from build123d import *

# Parameters (mm, degrees)
F0_W     = 7
F0_H     = 7
F0_W_2   = 4.5
F0_H_2   = 4.5
F1_DEPTH = 5
F2_W     = 7
F2_H     = 7
F3_DEPTH = 2
F4_W     = 1.960302
F4_H     = 7
F5_DEPTH = 15
F6_R     = 1.25
F7_DEPTH = 25


with BuildPart() as f1:
    # F0 (on Front) → F1 (new body)
    with BuildSketch(Plane.XZ):
        Rectangle(F0_W, F0_H)
        Rectangle(F0_W_2, F0_H_2, mode=Mode.SUBTRACT)
    extrude(amount=F1_DEPTH)

    # F2 (on face) → F3 (join)
    with BuildSketch(Plane.XZ.offset(5)):
        Rectangle(F2_W, F2_H)
    extrude(amount=F3_DEPTH)

    # F4 (on face) → F5 (join)
    with BuildSketch(Plane.XZ.offset(7)):
        Rectangle(F4_W, F4_H)
    extrude(amount=F5_DEPTH)

    # F6 (on face) → F7 (cut)
    with BuildSketch(Plane(origin=(-0.980151, 0, 0), x_dir=(0, -1, 0), z_dir=(-1, 0, 0))):
        with Locations((19, 0)):
            Circle(F6_R)
    extrude(amount=-F7_DEPTH, mode=Mode.SUBTRACT)


solid = f1.part
Work out the finished part from the listing and answer in its coordinate system (mm). A direction names the side the tool comes from. Give positions to 0.01 mm unless a question says otherwise; leave off trailing zeros. Write each loop counter-clockwise with the first axis right and the second up, starting at its lowest first coordinate (ties: lowest second). Pieces come first, ordered by that corner, then holes. Notation, with made-up numbers: (88, 46.25) - (147, 46.25) arc R28 ccw to (147, 64.25) - close; hole circle Ø9 at (34, -39.75). An arc over 180 degrees is marked (long way). One line per item, written item: value. Start each with the question number.
1. Find section C-C (x = 0.75). Write down the section's boundary in (y, z).
2. Find section D-D (z = 0). Write down the section's boundary in (x, y), then the cut area to 3 significant figures.
3. For a pull along X with two mould halves and no side action, classify faces 5 (the flat face through (0, -2, 2.25)), 6 (the cylindrical face through (-0.014, -20.155, -0.479)), 7 (the flat face through (3.5, -3, 0)) as +X half, -X half, draft (parallel to the pull), parting line (faces both ways), or undercut.
4. Find section B-B (y = -19). Write down the section's boundary in (x, z), then the cut area to 3 significant figures.
5. For faces 1 (the flat face through (0, -22, 0)), 2 (the flat face through (0.98, -14, 0)), 3 (the flat face through (0, -2, -2.25)), 4 (the flat face through (-2, -7, 0)), determine the directions among +Z, -Z, +X, -X, +Y, -Y from which every point of the face is accessible in a straight line to the end or side of a thin tool.
6. Given pin 1 (3 mm diameter, centred on x = 2, z = 0, fed in from -Y); pin 2 (1.5 mm diameter, centred on y = -13, z = 0, fed in from +X); pin 3 (2 mm diameter, centred on x = -2.5, z = 0, fed in from -Y), each flat-ended and moving along its own axis, determine where each tip first touches the part or whether it passes through.
7. Find section A-A (z = -1). Write down the section's boundary in (x, y), then the cut area to 3 significant figures.
8. Consider probe 1 along Z at (x, y) = (0.25, -19); probe 2 along Z at (x, y) = (1.75, -4.5); probe 3 along X at (y, z) = (-15.5, 2.5). Determine where each line is inside the solid, lowest interval first.
Geometry results:
1. outline: (-22, -3.5) - (0, -3.5) - (0, -2.25) - (-5, -2.25) - (-5, 2.25) - (0, 2.25) - (0, 3.5) - (-22, 3.5) - close; hole circle Ø2.5 at (-19, 0)
2. outline: (-3.5, -7) - (-0.98, -7) - (-0.98, -17.75) - (0.98, -17.75) - (0.98, -7) - (3.5, -7) - (3.5, 0) - (2.25, 0) - (2.25, -5) - (-2.25, -5) - (-2.25, 0) - (-3.5, 0) - close; (-0.98, -22) - (0.98, -22) - (0.98, -20.25) - (-0.98, -20.25) - close
2. area: 51.0 mm2
3. face 5: undercut
3. face 6: draft
3. face 7: +X half
4. outline: (-0.98, -3.5) - (0.98, -3.5) - (0.98, -1.25) - (-0.98, -1.25) - close; (-0.98, 1.25) - (0.98, 1.25) - (0.98, 3.5) - (-0.98, 3.5) - close
4. area: 8.82 mm2
5. face 1: +Z, -Z, +X, -X, -Y
5. face 2: +Z, -Z, +X, -Y
5. face 3: +Y
5. face 4: +Z, -Z, -X, -Y
6. pin 1: y = -22
6. pin 2: x = 0.98
6. pin 3: y = -7
7. outline: (-3.5, -7) - (-0.98, -7) - (-0.98, -18.25) - (0.98, -18.25) - (0.98, -7) - (3.5, -7) - (3.5, 0) - (2.25, 0) - (2.25, -5) - (-2.25, -5) - (-2.25, 0) - (-3.5, 0) - close; (-0.98, -22) - (0.98, -22) - (0.98, -19.75) - (-0.98, -19.75) - close
7. area: 53.0 mm2
8. probe 1: -3.5 to -1.25, 1.25 to 3.5
8. probe 2: -3.5 to -2.25, 2.25 to 3.5
8. probe 3: -0.98 to 0.98
